Input: part model. Units: mm. Frame: model coordinates. A direction names the side the tool comes from. Round coordinates to 2 decimals unless told otherwise and drop trailing zeros. Order: outer loops, then holes, each group sorted by start corner. A loop starts at its lowest first (then second) coordinate and runs counter-clockwise, first axis right, second up. Notation, with made-up numbers: (39.25, 66) -> (82.25, 66) arc R21 ccw to (82.25, 86) -> close; hole circle Ø10 at (45.5, 26). An arc over 180 degrees is marked (long way). Use a Markdown table: item, result.
from build123d import *

# Parameters (mm, degrees)
SKETCH_1_R          = 4
EXTRUDE_1_DEPTH     = 7
SKETCH_2_R          = 5
EXTRUDE_2_DEPTH     = 1
SKETCH_3_W          = 8
SKETCH_3_H          = 10
EXTRUDE_3_DEPTH     = 40
CUT_EXTRUDE_1_REACH = 11
SKETCH_4_R          = 2


with BuildPart() as part:
    # Эскиз1 → Бобышка-Вытянуть1 (new body)
    with BuildSketch(Plane.XY):
        Circle(SKETCH_1_R)
    extrude(amount=EXTRUDE_1_DEPTH)

    # Эскиз2 → Бобышка-Вытянуть2 (add)
    with BuildSketch(Plane.XY.offset(7)):
        Circle(SKETCH_2_R)
    extrude(amount=EXTRUDE_2_DEPTH)

    # Эскиз3 → Бобышка-Вытянуть3 (add)
    with BuildSketch(Plane.XY.offset(8)):
        Rectangle(SKETCH_3_W, SKETCH_3_H)
    extrude(amount=EXTRUDE_3_DEPTH)

    # Эскиз4 → Вырез-Вытянуть1 (cut, up to next)
    with BuildSketch(Plane.ZY.offset(4), mode=Mode.PRIVATE) as cut_extrude_1_sk1:
        with Locations((18, 0)):
            Circle(SKETCH_4_R)
    cut_extrude_1_tool1 = extrude(cut_extrude_1_sk1.sketch, amount=-CUT_EXTRUDE_1_REACH, mode=Mode.PRIVATE) & part.part
    add(cut_extrude_1_tool1.solids().sort_by_distance((-4, 0, 18))[0], mode=Mode.SUBTRACT)
    # Эскиз4 → Вырез-Вытянуть1 (cut, up to next)
    with BuildSketch(Plane.ZY.offset(4), mode=Mode.PRIVATE) as cut_extrude_1_sk2:
        with Locations((38, 0)):
            Circle(SKETCH_4_R)
    cut_extrude_1_tool2 = extrude(cut_extrude_1_sk2.sketch, amount=-CUT_EXTRUDE_1_REACH, mode=Mode.PRIVATE) & part.part
    add(cut_extrude_1_tool2.solids().sort_by_distance((-4, 0, 38))[0], mode=Mode.SUBTRACT)


solid = part.part
1) Cut plane D-D on z = 44.5. Return loops of the section in (x, y).
Answer key:
| item | result |
|---|---|
| outline | (-4, -5) -> (4, -5) -> (4, 5) -> (-4, 5) -> close |
2) Set-up query: faces 1 (the face through (-3, 4.5, 8)), 2 (the face through (-1.08, -4.88, 7.49)), 3 (the face through (4, 0, 28)). Return all of +Z, -Z, +X, -X, +Y, -Y with unobstructed straight access to the full face (end or side cutting, diameter ignored); none if empty.
Answer key:
| item | result |
|---|---|
| face 1 | -Z, -X, +Y |
| face 2 | -Z |
| face 3 | +Z, +X, +Y, -Y |
3) Ray query, probe 1 along Y at (x, z) = (0.25, 38); probe 2 along Z at (x, y) = (2, 1.5); probe 3 along X at (y, z) = (-4.5, 20). Return the intervals inside material, ascending.
Answer key:
| item | result |
|---|---|
| probe 1 | y = -5 to -2, 2 to 5 |
| probe 2 | z = 0 to 16.68, 19.32 to 36.68, 39.32 to 48 |
| probe 3 | x = -4 to 4 |
4) Cut plane B-B on z = 38. Return loops of the section in (x, y), and give its area (3 significant figures).
Answer key:
| item | result |
|---|---|
| outline | (-4, -5) -> (4, -5) -> (4, -2) -> (-4, -2) -> close; (-4, 2) -> (4, 2) -> (4, 5) -> (-4, 5) -> close |
| area | 48.0 mm^2 |
5) Contact query for flat-ended pins moving along their axis: P1, Ø4.5, axis at y = 0, z = 18, coming from the -X side; P2, Ø3.5, axis at y = 0, z = 38, coming from the +X side; P3, Ø1, axis at x = -2.5, y = -4, coming from the -Z side; P4, Ø5, axis at y = -1.5, z = 27.5, coming from the +X side. Output: stop coordinate, or through.
Answer key:
| item | result |
|---|---|
| P1 | stops at x = -4 |
| P2 | passes through |
| P3 | stops at z = 7 |
| P4 | stops at x = 4 |
6) Draft query along Z for faces 4 (the face through (-3, -4.5, 8)), 5 (the face through (0, 0, 36)), 6 (the face through (-4, 0, 28)), 7 (the face through (-4.4, 0, 8)). Return one class per face: released by +Z, released by -Z, zero draft, split by the parting line, or undercut.
Answer key:
| item | result |
|---|---|
| face 4 | released by -Z |
| face 5 | undercut |
| face 6 | zero draft |
| face 7 | released by +Z |
7) Cut plane C-C on x = 1.25. Return loops of the section in (y, z).
Answer key:
| item | result |
|---|---|
| outline | (-5, 8) -> (-4.84, 8) -> (-4.84, 7) -> (-3.8, 7) -> (-3.8, 0) -> (3.8, 0) -> (3.8, 7) -> (4.84, 7) -> (4.84, 8) -> (5, 8) -> (5, 48) -> (-5, 48) -> close; hole circle Ø4 at (0, 18); hole circle Ø4 at (0, 38) |
8) Cut plane A-A on y = 0. Return loops of the section in (x, z).
Answer key:
| item | result |
|---|---|
| outline | (-5, 7) -> (-4, 7) -> (-4, 0) -> (4, 0) -> (4, 7) -> (5, 7) -> (5, 8) -> (4, 8) -> (4, 16) -> (-4, 16) -> (-4, 8) -> (-5, 8) -> close; (-4, 20) -> (4, 20) -> (4, 36) -> (-4, 36) -> close; (-4, 40) -> (4, 40) -> (4, 48) -> (-4, 48) -> close |
